from build123d import *

# Parameters (mm, degrees)
SKETCH1_R           = 5
SKETCH1_R_2         = 3
BOSS_EXTRUDE1_DEPTH = 30
CUT_EXTRUDE1_START  = -10
CUT_EXTRUDE1_DEPTH  = 11


with BuildPart() as part:
    # Sketch1 → Boss-Extrude1 (new body, symmetric)
    with BuildSketch(Plane.XY):
        Circle(SKETCH1_R)
        Circle(SKETCH1_R_2, mode=Mode.SUBTRACT)
    extrude(amount=BOSS_EXTRUDE1_DEPTH, both=True)

    # Sketch4 → Cut-Extrude1 (cut)
    with BuildSketch(Plane.XY.offset(30).offset(CUT_EXTRUDE1_START)):
        with BuildLine():
            Line((-2.179449472, 4.5), (2.179449472, 4.5))
            ThreePointArc((2.179449472, 4.5), (0, 5), (-2.179449472, 4.5))
        make_face()
    cut_extrude1 = extrude(amount=CUT_EXTRUDE1_DEPTH, mode=Mode.SUBTRACT)

    # Mirror3: Cut-Extrude1 across plane
    add(cut_extrude1.mirror(Plane.XY), mode=Mode.SUBTRACT)


solid = part.part
Geometry check sheet. Reference: the model listing, model coordinates, mm. A direction names the side the tool comes from. Coordinates: 2 decimals unless noted, no trailing zeros. Order: outer loops, then holes, each group sorted by start corner. A loop starts at its lowest first (then second) coordinate and runs counter-clockwise, first axis right, second up. Notation, with made-up numbers: (53, -6.5) -> (84, -6.5) arc R8 cw to (84, 2.5) -> close; hole circle Ø11 at (88.25, 80). An arc over 180 degrees is marked (long way). Use a Markdown table: item, result. Add a question column.
1. Set-up check for faces 4 (the face through (0, 4.5, -25)), 5 (the face through (0, 4.5, 25)), 6 (the face through (2.2, -2.3, 30)): record each of +Z, -Z, +X, -X, +Y, -Y from which the full face is reachable in a straight line by a thin tool's end or side.
2. Cross-section at B-B (x = 0). Enter the section's corners in (y, z), and give its area (3 significant figures).
3. Go/stop test with flat-tipped pins: pin 1 Ø1.3 at (x, z) = (0, -25) entering from +Y; pin 2 Ø1 at (x, z) = (-3, 14.5) entering from -Y; pin 3 Ø3 at (x, z) = (-3.5, -13) entering from -Y. Record where each tip stops, or that it passes through.
4. Cross-section at C-C (z = -1.5). Enter the section's corners in (x, y).
5. Material ranges on L1, parallel to Y at x = 0, z = 17; L2, parallel to Y at x = -0.25, z = -26.5; L3, parallel to X at y = 1.75, z = -2.5, recorded low to high.
6. Cross-section at D-D (y = -4). Enter the section's corners in (x, z).
7. Cross-section at A-A (y = 0). Enter the section's corners in (x, z), and give its area (3 significant figures).
8. Mould release check, pull along X, two halves, no side actions. Record for faces 1 (the face through (-3, 0, 0)), 2 (the face through (2.2, -2.3, -30)), 3 (the face through (-1.08, -4.88, 0.42)): pulls with the +X half, pulls with the -X half, needs draft (parallel to the pull), parting line crosses it, or undercut.
Filled sheet:
| question | item | result |
|---|---|---|
| 1 | face 4 | -Z, +X, -X, +Y |
| 1 | face 5 | +Z, +X, -X, +Y |
| 1 | face 6 | +Z, +X, -X, +Y, -Y |
| 2 | outline | (-5, -30) -> (-3, -30) -> (-3, 30) -> (-5, 30) -> close; (3, -30) -> (4.5, -30) -> (4.5, -20) -> (5, -20) -> (5, 20) -> (4.5, 20) -> (4.5, 30) -> (3, 30) -> close |
| 2 | area | 230 mm2 |
| 3 | pin 1 | y = 4.5 |
| 3 | pin 2 | y = -4.33 |
| 3 | pin 3 | y = -4.58 |
| 4 | outline | circle Ø10 at (0, 0); hole circle Ø6 at (0, 0) |
| 5 | L1 | -5 to -3, 3 to 5 |
| 5 | L2 | -4.99 to -2.99, 2.99 to 4.5 |
| 5 | L3 | -4.68 to -2.44, 2.44 to 4.68 |
| 6 | outline | (-3, -30) -> (3, -30) -> (3, 30) -> (-3, 30) -> close |
| 7 | outline | (-5, -30) -> (-3, -30) -> (-3, 30) -> (-5, 30) -> close; (3, -30) -> (5, -30) -> (5, 30) -> (3, 30) -> close |
| 7 | area | 240 mm2 |
| 8 | face 1 | undercut |
| 8 | face 2 | needs draft |
| 8 | face 3 | parting line crosses it |
